Can you work these out from the model? Positions are in its coordinate system, mm. A direction names the side the tool comes from. Coordinates: 2 decimals unless noted, no trailing zeros. Order: outer loops, then holes, each group sorted by start corner. A loop starts at its lowest first (then second) coordinate and runs counter-clockwise, first axis right, second up. Notation, with made-up numbers: M 11,39.5 L 38,39.5 A7 cw 38,47.5 Z; hole C -30,-5.75 d4. An arc over 180 degrees is marked long. Answer as a JSON object with one key per item and string values.
from build123d import *

# Parameters (mm, degrees)
SKETCH1_W           = 81
SKETCH1_H           = 41
BOSS_EXTRUDE1_DEPTH = 6
SKETCH5_W           = 75
SKETCH5_H           = 35
CUT_EXTRUDE1_DEPTH  = 1.43
SKETCH8_R           = 2.1
SKETCH8_R_2         = 4
CUT_EXTRUDE2_DEPTH  = 46.787552894
SKETCH9_R           = 2.75
CUT_EXTRUDE3_DEPTH  = 1.5
FILLET1_R           = 1
SKETCH10_W          = 4.57
SKETCH10_H          = 24
BOSS_EXTRUDE2_DEPTH = 12
SKETCH12_W          = 4.57
SKETCH12_H          = 24
BOSS_EXTRUDE3_DEPTH = 12
SKETCH13_R          = 2.1
CUT_EXTRUDE4_DEPTH  = 57.545423334
SKETCH14_W          = 3
SKETCH14_H          = 15
SKETCH14_H_2        = 6
BOSS_EXTRUDE4_DEPTH = 8
SKETCH15_W          = 10.5
SKETCH15_H          = 4
CUT_EXTRUDE5_DEPTH  = 71.75485849


with BuildPart() as part:
    # Sketch1 → Boss-Extrude1 (new body)
    with BuildSketch(Plane.XY):
        Rectangle(SKETCH1_W, SKETCH1_H)
    extrude(amount=BOSS_EXTRUDE1_DEPTH)

    # Sketch5 → Cut-Extrude1 (cut)
    with BuildSketch(Plane(origin=(0, 0, 0), x_dir=(-1, 0, 0), z_dir=(0, 0, -1))):
        Rectangle(SKETCH5_W, SKETCH5_H)
    extrude(amount=-CUT_EXTRUDE1_DEPTH, mode=Mode.SUBTRACT)

    # Sketch8 → Cut-Extrude2 (cut, through all)
    with BuildSketch(Plane.XY.offset(6)):
        with Locations((26.9, 0.5)):
            Circle(SKETCH8_R)
        with Locations((20.55, 6.849637785)):
            Circle(SKETCH8_R)
        with Locations((7.85, 6.849637785)):
            Circle(SKETCH8_R)
        with Locations((7.85, -5.849637785)):
            Circle(SKETCH8_R)
        with Locations((20.55, -5.849637785)):
            Circle(SKETCH8_R)
        with Locations((1.5, 0.5)):
            Circle(SKETCH8_R)
        with Locations((-4.85, 6.849637785)):
            Circle(SKETCH8_R)
        with Locations((-4.85, -5.849637785)):
            Circle(SKETCH8_R)
        with Locations((-11.2, 0.5)):
            Circle(SKETCH8_R)
        with Locations((-17.55, 6.849637785)):
            Circle(SKETCH8_R)
        with Locations((-17.55, -5.849637785)):
            Circle(SKETCH8_R)
        with Locations((14.2, 0.5)):
            Circle(SKETCH8_R_2)
    extrude(amount=-CUT_EXTRUDE2_DEPTH, mode=Mode.SUBTRACT)

    # Sketch9 → Cut-Extrude3 (cut)
    with BuildSketch(Plane(origin=(0, 20.5, 0), x_dir=(1, 0, 0), z_dir=(0, 1, 0))):
        with Locations((6.35, -1.35)):
            Circle(SKETCH9_R)
        with Locations((-6.35, -1.35)):
            Circle(SKETCH9_R)
    extrude(amount=-CUT_EXTRUDE3_DEPTH, mode=Mode.SUBTRACT)

    # Fillet1
    fillet1_edges = [part.edges().sort_by_distance(p)[0] for p in [
        (-8.74582971, 19.75, 0),
        (-3.95417029, 19.75, 0),
        (3.95417029, 19.75, 0),
        (8.74582971, 19.75, 0),
    ]]
    fillet(fillet1_edges, radius=FILLET1_R)

    # Sketch10 → Boss-Extrude2 (add)
    with BuildSketch(Plane.ZY.offset(40.5)):
        with Locations((2.285, -8.5)):
            Rectangle(SKETCH10_W, SKETCH10_H)
    extrude(amount=BOSS_EXTRUDE2_DEPTH)

    # Sketch12 → Boss-Extrude3 (add)
    with BuildSketch(Plane(origin=(40.5, 0, 0), x_dir=(0, 0, -1), z_dir=(1, 0, 0))):
        with Locations((-2.285, -8.5)):
            Rectangle(SKETCH12_W, SKETCH12_H)
    extrude(amount=BOSS_EXTRUDE3_DEPTH)

    # Sketch13 → Cut-Extrude4 (cut, through all)
    with BuildSketch(Plane.XY.offset(4.57)):
        with Locations((-46.5, -3.5)):
            Circle(SKETCH13_R)
        with Locations((-46.5, -13.5)):
            Circle(SKETCH13_R)
        with Locations((46.5, -3.5)):
            Circle(SKETCH13_R)
        with Locations((46.5, -13.5)):
            Circle(SKETCH13_R)
    extrude(amount=-CUT_EXTRUDE4_DEPTH, mode=Mode.SUBTRACT)

    # Sketch14 → Boss-Extrude4 (add)
    with BuildSketch(Plane.XZ.offset(20.5)):
        with Locations((9, -7.5)):
            Rectangle(SKETCH14_W, SKETCH14_H)
        with Locations((9, 3)):
            Rectangle(SKETCH14_W, SKETCH14_H_2)
    extrude(amount=BOSS_EXTRUDE4_DEPTH)

    # Sketch15 → Cut-Extrude5 (cut, through all)
    with BuildSketch(Plane(origin=(10.5, 0, 0), x_dir=(0, 0, -1), z_dir=(1, 0, 0))):
        with Locations((4.5, -24.5)):
            Rectangle(SKETCH15_W, SKETCH15_H)
    extrude(amount=-CUT_EXTRUDE5_DEPTH, mode=Mode.SUBTRACT)


solid = part.part
Item 1: I'm going to push flat-ended pins straight in: pin 1 (2.5 mm diameter, centred on x = 7.85, y = -5.85, fed in from -Z); pin 2 (9 mm diameter, centred on y = -26, z = -5, fed in from -X); pin 3 (2.5 mm diameter, centred on x = 9, z = -8, fed in from +Y); pin 4 (9 mm diameter, centred on y = -26.5, z = -8.5, fed in from +X). Where does each tip first touch, or does it pass through?
Answers follow:
{"pin 1": "passes through", "pin 2": "stops at x = 7.5", "pin 3": "stops at y = -20.5", "pin 4": "stops at x = 10.5"}
Item 2: I want a section at D-D, the plane x = 32.5. Write out the boundary of the cut face in (y, z), plus the area to 3 significant figures.
Answers follow:
{"outline": "M -20.5,0 L -17.5,0 L -17.5,1.43 L 17.5,1.43 L 17.5,0 L 20.5,0 L 20.5,6 L -20.5,6 Z", "area": "196 mm^2"}
Item 3: I want a section at A-A, the plane z = -8. Write out the boundary of the cut face in (x, y).
Answers follow:
{"outline": "M 7.5,-28.5 L 10.5,-28.5 L 10.5,-26.5 L 7.5,-26.5 Z; M 7.5,-22.5 L 10.5,-22.5 L 10.5,-20.5 L 7.5,-20.5 Z"}
Item 4: Please list where these lines run through material, in increasing order: line 1 (Y direction, x = -17.55, z = 3.4); line 2 (Y direction, x = 46.5, z = 1); line 3 (Y direction, x = 1.5, z = 1.5).
Answers follow:
{"line 1": "y = -20.5 to -7.95, -3.75 to 4.75, 8.95 to 20.5", "line 2": "y = -20.5 to -15.6, -11.4 to -5.6, -1.4 to 3.5", "line 3": "y = -20.5 to -1.6, 2.6 to 20.5"}
Item 5: Which directions (+Z, -Z, +X, -X, +Y, -Y) give clear straight access to the entire face, cutting with the end or side of a thin tool? Please do faces 4 (the flat face through (9, -25, -9.75)), 5 (the flat face through (1, -4, 1.43)), 6 (the flat face through (-23, -20.5, 3)), 7 (the flat face through (46, -9, 4.57)).
Answers follow:
{"face 4": "+X, -X", "face 5": "-Z", "face 6": "+Z, -Z, -X, -Y", "face 7": "+Z, +X, +Y, -Y"}
Item 6: I want a section at C-C, the plane y = 0.5. Write out the boundary of the cut face in (x, z), plus the area to 3 significant figures.
Answers follow:
{"outline": "M -52.5,0 L -37.5,0 L -37.5,1.43 L -13.3,1.43 L -13.3,6 L -40.5,6 L -40.5,4.57 L -52.5,4.57 Z; M -9.1,1.43 L -0.6,1.43 L -0.6,6 L -9.1,6 Z; M 3.6,1.43 L 10.2,1.43 L 10.2,6 L 3.6,6 Z; M 18.2,1.43 L 24.8,1.43 L 24.8,6 L 18.2,6 Z; M 29,1.43 L 37.5,1.43 L 37.5,0 L 52.5,0 L 52.5,4.57 L 40.5,4.57 L 40.5,6 L 29,6 Z", "area": "394 mm^2"}
Item 7: If we mould it in two halves opening along X, with no side actions, what happens to faces 1 (the flat face through (7.5, -22, -4)), 2 (the cylindrical face through (-19.216, 5.572, 3.747)), 3 (the flat face through (9, -25, 0.75))? For each: pulls with the +X half, pulls with the -X half, needs draft (parallel to the pull), parting line crosses it, or undercut.
Answers follow:
{"face 1": "pulls with the -X half", "face 2": "undercut", "face 3": "needs draft"}
Item 8: I want a section at B-B, the plane x = 1.5. Write out the boundary of the cut face in (y, z), plus the area to 3 significant figures.
Answers follow:
{"outline": "M -20.5,0 L -17.5,0 L -17.5,1.43 L -1.6,1.43 L -1.6,6 L -20.5,6 Z; M 2.6,1.43 L 17.5,1.43 L 17.5,0 L 20.5,0 L 20.5,6 L 2.6,6 Z", "area": "177 mm^2"}
